For this review, take the finished solid that the model builds, in its own axes (mm). Face numbers are marked on the shaded views. Coordinates: 2 decimals unless noted, no trailing zeros. Order: outer loops, then holes, each group sorted by start corner. A loop starts at its lowest first (then second) coordinate and runs counter-clockwise, first axis right, second up. Notation, with made-up numbers: (30, -1.5) - (39, -1.5) arc R22 ccw to (39, 34.5) - close; hole circle Ø7 at (4, 50). An arc over 180 degrees is marked (long way). One line per item, written item: value. Start each with the question number.
(1) Clearance check with flat-ended pins moving along their axes: pin 1 (0.8 mm diameter, centred on x = 37.5, z = 3.5, fed in from -Y); pin 2 (24.5 mm diameter, centred on x = -22.5, z = -38.5, fed in from +Y); pin 3 (9.5 mm diameter, centred on x = -20, z = -27.5, fed in from -Y). State where each tip first meets the part, or that it passes through.
(2) Consider section A-A on y = 4. Write out the cut boundary in (x, z).
(3) Consider section B-B on x = 38. Write out the cut boundary in (y, z).
(4) Mouldability with a two-part tool opening along Z and no side actions: class the marked faces 1 and 2 as released by +Z, released by -Z, zero draft, split by the parting line, or undercut.
(5) To check wall thickness, follow line 1 along Z through (x, y) = (0, 2); line 2 along Z through (x, y) = (-6, 3); line 3 along X through (y, z) = (1.5, -50). State the ranges of each line that lie inside material, in increasing order.
Autodesk Inventor part; units mm, degrees
ref_plane "Work Plane1" through (5, 0, 0) normal (1, 0, 0) x (0, 1, 0)
ref_plane "YZ Plane" through (0, 0, 0) normal (1, 0, 0) x (0, 1, 0)
ref_plane "XZ Plane" through (0, 0, 0) normal (0, 1, 0) x (-1, 0, 0)
sketch "Sketch1" plane through (0, 0, 0) normal (0, 1, 0) x (-1, 0, 0)
  circle A0 centre (0, 0) radius 2.5
  circle A1 centre (0, 0) radius 63.5
  circle A2 centre (0, 0) radius 5
  dimension "d1" = 127
  dimension "d4" = 10
extrude "Extrusion1" add sketch "Sketch1" along normal blind 7 contours A2
ref_plane "Work Plane1" through (5, 0, 0) normal (1, 0, 0) x (0, 1, 0)
sketch "Sketch3" plane through (5, 0, 0) normal (1, 0, 0) x (0, 1, 0)
  line L0 (7, -5) -> (7, 5)
  arc A0 (6.5749, -3.5929) -> (0.5749, 2.4071) centre (-24.5498, -28.7176) ccw
  line L1 (0.5749, 2.4071) -> (0.5749, 3.9071)
  arc A1 (0.5749, 3.9071) -> (6.5749, -2.0929) centre (22.8832, 20.2155) ccw
  line L2 (6.5749, -2.0929) -> (6.5749, -3.5929)
  point P0 (0, 0)
  dimension "d13" = 40
  dimension "d15" = 1.5
extrude "Extrusion3" add sketch "Sketch3" against normal blind 2 and the other way blind 58.5
fillet "Fillet2" radius 0.25 4 edges at (5, 7, 0) (5, 0, 0) (2.5, 7, 0) (2.5, 0, 0)
pattern_circular "Circular Pattern1" count 3 over 360 about axis through (0, 0, 0) along (0, 1, 0) of "Extrusion3"
properties part number "DAL T5040"
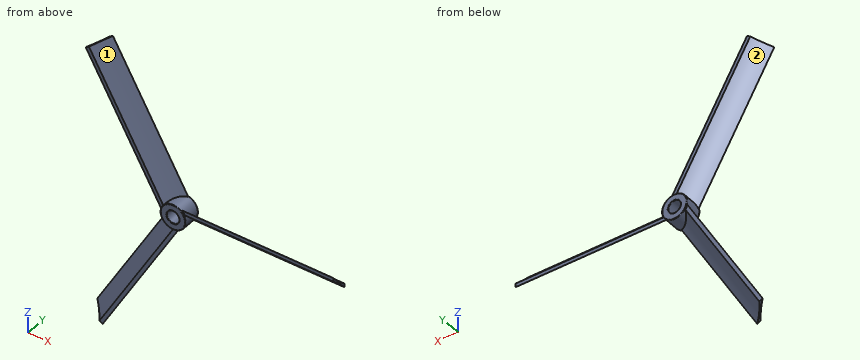
Geometry check:
1. pin 1: stops at y = 0.57
1. pin 2: stops at y = 6.57
1. pin 3: stops at y = 2.02
2. outline: (-32.36, -54.64) - (-31.72, -55.01) - (-2.47, -4.35) arc R5 ccw to (4.95, -0.7) - (63.5, -0.7) - (63.5, 0.04) - (5, 0.04) arc R5 ccw to (-1.87, 4.64) - (-31.14, 55.34) - (-31.78, 54.97) - (-2.53, 4.31) arc R5 ccw to (-3.08, -3.94) - close; hole circle Ø5 at (0, 0)
3. outline: (0.57, 2.41) arc R40 cw to (6.57, -3.59) - (6.57, -2.09) arc R27.63 cw to (0.57, 3.91) - close
4. face 1: released by +Z
4. face 2: undercut
5. line 1: z = -5 to -2.5, 2.5 to 5
5. line 2: z = -12.44 to -10.96, 8.34 to 9.83
5. line 3: x = -26.98 to -25.74
